Geometry: see drawing. Coordinates: mm, zero at the bounding-box minimum. A direction names the side the tool comes from. Round coordinates to 2 decimals unless told otherwise and drop trailing zeros. Order: outer loops, then holes, each group sorted by start corner. A loop starts at its lowest first (then second) coordinate and runs counter-clockwise, first axis right, second up. Notation, with made-up numbers: (86, 89) -> (116, 89) arc R26 cw to (116, 126) -> close; hole circle Ø5 at (29.25, 8). An arc over 180 degrees is marked (long way). Use a Markdown table: item, result.
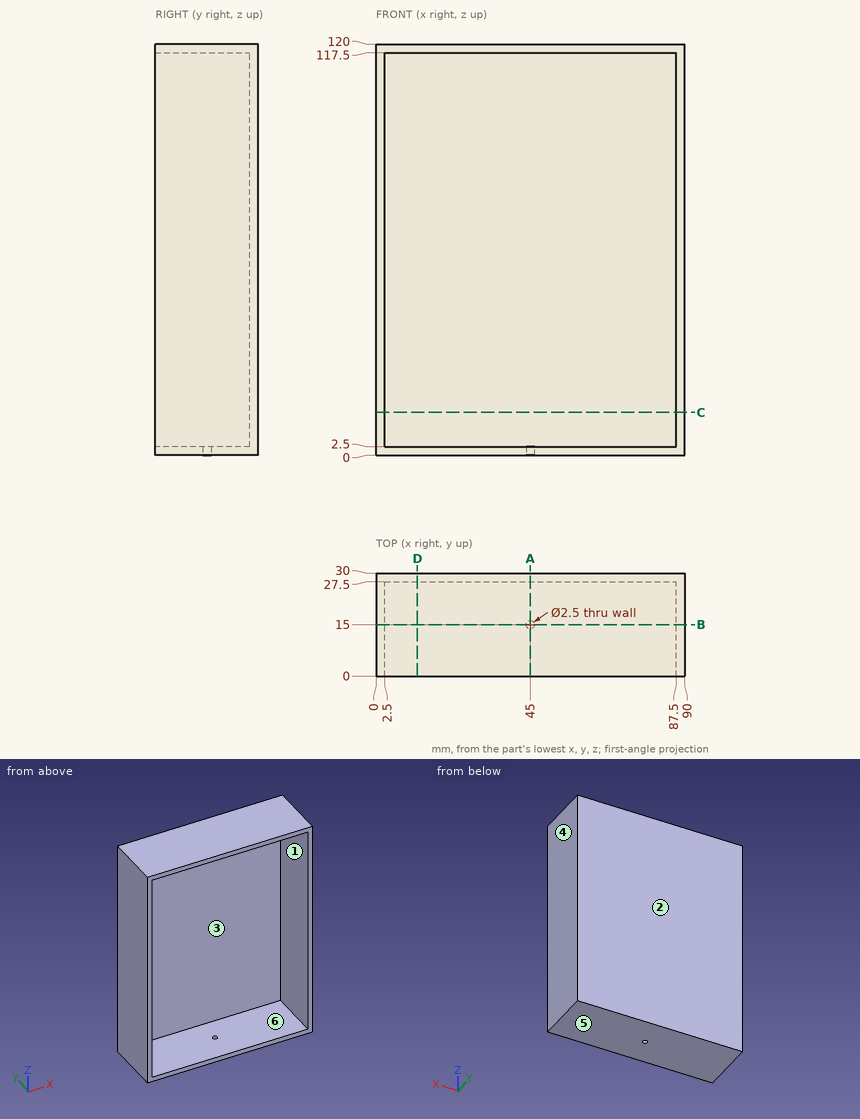
1) Cut plane C-C on z = 12.5. Return loops of the section in (x, y), and give its area (4 significant figures).
Answer key:
| item | result |
|---|---|
| outline | (0, 0) -> (2.5, 0) -> (2.5, 27.5) -> (87.5, 27.5) -> (87.5, 0) -> (90, 0) -> (90, 30) -> (0, 30) -> close |
| area | 362.5 mm^2 |
2) Cut plane A-A on x = 45. Return loops of the section in (y, z).
Answer key:
| item | result |
|---|---|
| outline | (0, 0) -> (13.75, 0) -> (13.75, 2.5) -> (0, 2.5) -> close; (0, 117.5) -> (27.5, 117.5) -> (27.5, 2.5) -> (16.25, 2.5) -> (16.25, 0) -> (30, 0) -> (30, 120) -> (0, 120) -> close |
3) Set-up query: the marked faces 1 and 2. Return all of +Z, -Z, +X, -X, +Y, -Y with unobstructed straight access to the full face (end or side cutting, diameter ignored); none if empty.
Answer key:
| item | result |
|---|---|
| face 1 | -Y |
| face 2 | +Z, -Z, +X, -X, +Y |
4) Ray query, probe 1 along Z at (x, y) = (15.5, 13.5); probe 2 along X at (y, z) = (25.5, 35); probe 3 along Y at (x, z) = (45, 1.7). Return the intervals inside material, ascending.
Answer key:
| item | result |
|---|---|
| probe 1 | z = 0 to 2.5, 117.5 to 120 |
| probe 2 | x = 0 to 2.5, 87.5 to 90 |
| probe 3 | y = 0 to 13.75, 16.25 to 30 |
5) Draft query along Z for the marked faces 3, 4, 5 and 6. Return one class per face: released by +Z, released by -Z, zero draft, split by the parting line, or undercut.
Answer key:
| item | result |
|---|---|
| face 3 | undercut |
| face 4 | zero draft |
| face 5 | released by -Z |
| face 6 | undercut |
6) Cut plane B-B on y = 15. Return loops of the section in (x, z), and give its area (3 significant figures).
Answer key:
| item | result |
|---|---|
| outline | (0, 0) -> (43.75, 0) -> (43.75, 2.5) -> (2.5, 2.5) -> (2.5, 117.5) -> (87.5, 117.5) -> (87.5, 2.5) -> (46.25, 2.5) -> (46.25, 0) -> (90, 0) -> (90, 120) -> (0, 120) -> close |
| area | 1,020 mm^2 |
7) Cut plane D-D on x = 12. Return loops of the section in (y, z), and give its area (4 significant figures).
Answer key:
| item | result |
|---|---|
| outline | (0, 0) -> (30, 0) -> (30, 120) -> (0, 120) -> (0, 117.5) -> (27.5, 117.5) -> (27.5, 2.5) -> (0, 2.5) -> close |
| area | 437.5 mm^2 |
8) Contact query for a flat-ended pin moving along its axis: P1, Ø5, axis at x = 56, z = 96, coming from the -Y side. Output: stop coordinate, or through.
Answer key:
| item | result |
|---|---|
| P1 | stops at y = 27.5 |
